Part model, mm, in its own coordinate system. Face numbers are marked on the shaded views. A direction names the side the tool comes from. Round coordinates to 2 decimals unless told otherwise and drop trailing zeros. Write each loop counter-clockwise with the first axis right and the second up, starting at its lowest first coordinate (ties: lowest second). Pieces come first, ordered by that corner, then holes.
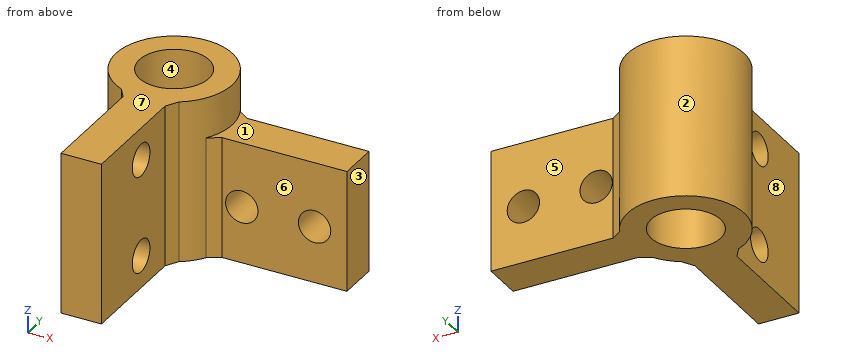
```python
from build123d import *

# Parameters (mm, degrees)
CYLINDER036_R          = 4.3
CYLINDER036_DEPTH      = 200
CYLINDER043_R          = 2
CYLINDER043_DEPTH      = 10
CYLINDER043_ROLL_ANGLE = 90
CYLINDER042_R          = 2
CYLINDER042_DEPTH      = 10
CYLINDER042_ROLL_ANGLE = 90
BOX010_W               = 24
BOX010_H               = 5
BOX010_DEPTH           = 15
CYLINDER044_R          = 2
CYLINDER044_DEPTH      = 10
CYLINDER045_R          = 2
CYLINDER045_DEPTH      = 10
BOX011_W               = 19
BOX011_H               = 5
BOX011_DEPTH           = 20
BOX011_PLACEMENT_ANGLE = -90
CYLINDER041_R          = 7.2
CYLINDER041_DEPTH      = 20
CHAMFER006_SIZE        = 1


with BuildPart() as cilindro033:
    # Cylinder036 → Cylinder036 (new body)
    with BuildSketch(Plane(origin=(57, -40, -29), x_dir=(1, 0, 0), z_dir=(0, 0, 1))):
        Circle(CYLINDER036_R)
    extrude(amount=CYLINDER036_DEPTH)


with BuildPart() as cilindro040:
    # Cylinder043 → Cylinder043 (new body)
    with BuildSketch(Plane.XY):
        Circle(CYLINDER043_R)
    extrude(amount=CYLINDER043_DEPTH)


with BuildPart() as cilindro040_1:
    # Cylinder043 roll: moved
    add(cilindro040.part.rotate(Axis((0, 0, 0), (1, 0, 0)), CYLINDER043_ROLL_ANGLE))


with BuildPart() as cilindro040_2:
    # Cylinder043 placement: moved
    add(cilindro040_1.part.moved(Location((76, -37, 30))))


with BuildPart() as fusion007:
    # Cylinder042 → Cylinder042 (new body)
    with BuildSketch(Plane.XY):
        Circle(CYLINDER042_R)
    extrude(amount=CYLINDER042_DEPTH)


with BuildPart() as fusion007_1:
    # Cylinder042 roll: moved
    add(fusion007.part.rotate(Axis((0, 0, 0), (1, 0, 0)), CYLINDER042_ROLL_ANGLE))


with BuildPart() as fusion007_2:
    # Cylinder042 placement: moved
    add(fusion007_1.part.moved(Location((67, -37, 30))))

    # Fusion007: union Cilindro040
    add(cilindro040_2.part)


with BuildPart() as cut032:
    # Box010 → Box010 (new body)
    with BuildSketch(Plane(origin=(56, -43, 23), x_dir=(1, 0, 0), z_dir=(0, 0, 1))):
        with Locations((12, 2.5)):
            Rectangle(BOX010_W, BOX010_H)
    extrude(amount=BOX010_DEPTH)

    # Cut032: cut Fusion007
    add(fusion007_2.part, mode=Mode.SUBTRACT)


with BuildPart() as cut032_1:
    # Cut032 placement: moved
    add(cut032.part.moved(Location((0, 0, -2))))


with BuildPart() as cilindro041:
    # Cylinder044 → Cylinder044 (new body)
    with BuildSketch(Plane(origin=(63, -53, 25), x_dir=(0, -1, 0), z_dir=(-1, 0, 0))):
        Circle(CYLINDER044_R)
    extrude(amount=CYLINDER044_DEPTH)


with BuildPart() as fusion008:
    # Cylinder045 → Cylinder045 (new body)
    with BuildSketch(Plane(origin=(63, -53, 37), x_dir=(0, -1, 0), z_dir=(-1, 0, 0))):
        Circle(CYLINDER045_R)
    extrude(amount=CYLINDER045_DEPTH)

    # Fusion008: union Cilindro041
    add(cilindro041.part)


with BuildPart() as cut033:
    # Box011 → Box011 (new body)
    with BuildSketch(Plane.XY):
        with Locations((9.5, 2.5)):
            Rectangle(BOX011_W, BOX011_H)
    extrude(amount=BOX011_DEPTH)


with BuildPart() as cut033_1:
    # Box011 placement: moved
    add(cut033.part.moved(Location((55, -43, 21))).rotate(Axis((55, -43, 21), (0, 0, 1)), BOX011_PLACEMENT_ANGLE))

    # Cut033: cut Fusion008
    add(fusion008.part, mode=Mode.SUBTRACT)


with BuildPart() as rodamiento_lineal:
    # Cylinder041 → Cylinder041 (new body)
    with BuildSketch(Plane(origin=(57, -40, 21), x_dir=(1, 0, 0), z_dir=(0, 0, 1))):
        Circle(CYLINDER041_R)
    extrude(amount=CYLINDER041_DEPTH)

    # Fusion009: union Cut032, Cut033
    add(cut032_1.part)
    add(cut033_1.part)

    # Chamfer006
    chamfer006_edges = [rodamiento_lineal.edges().sort_by_distance(p)[0] for p in [
        (63.916647, -38, 28.5),
        (63.545227, -43, 28.5),
        (55, -46.916647, 31),
        (60, -46.545227, 31),
    ]]
    chamfer(chamfer006_edges, length=CHAMFER006_SIZE)

    # Cut034: cut Cilindro033
    add(cilindro033.part, mode=Mode.SUBTRACT)


solid = rodamiento_lineal.part
```
Q1. Drop flat-ended pins along their axis: pin 1 (6 mm diameter, centred on x = 65, y = -53.5, fed in from -Z); pin 2 (7.5 mm diameter, centred on x = 71.5, z = 26.5, fed in from -Y); pin 3 (7.5 mm diameter, centred on x = 69.5, y = -41.5, fed in from +Z); pin 4 (5 mm diameter, centred on y = -53, z = 25, fed in from -X). Give the stop position or say it passes through.
Values follow:
pin 1: passes through
pin 2: stops at y = -43
pin 3: stops at z = 36
pin 4: stops at x = 55
Q2. Cut at A-A on y = -53. Write the cut outline in (x, z), plus the area to 3 significant figures.
Values follow:
outline: (55, 21) - (60, 21) - (60, 23) - (55, 23) - close; (55, 27) - (60, 27) - (60, 35) - (55, 35) - close; (55, 39) - (60, 39) - (60, 41) - (55, 41) - close
area: 60.0 mm2
Q3. Cut at B-B on x = 57. Write the cut outline in (y, z).
Values follow:
outline: (-62, 21) - (-44.3, 21) - (-44.3, 41) - (-62, 41) - close; (-35.7, 21) - (-32.8, 21) - (-32.8, 41) - (-35.7, 41) - close; hole circle Ø4 at (-53, 25); hole circle Ø4 at (-53, 37)
Q4. Cut at D-D on x = 76. Write the cut outline in (y, z), plus the area to 3 significant figures.
Values follow:
outline: (-43, 21) - (-38, 21) - (-38, 26) - (-43, 26) - close; (-43, 30) - (-38, 30) - (-38, 36) - (-43, 36) - close
area: 55.0 mm2
Q5. Which spindle directions (+Z, -Z, +X, -X, +Y, -Y) get a long thin tool onto all of the face, cutting with end or side? Do the marked faces 5, 6, 7 and 8. Say none if no direction does.
Values follow:
face 5: +Z, -Z, +X, +Y
face 6: +Z, -Z, +X, -Y
face 7: +Z, +X, -X, +Y, -Y
face 8: +Z, -Z, -X, -Y
Q6. Mould opens along X. For the marked faces 1, 2, 3 and 4 say: +X half, -X half, draft (parallel to the pull), parting line (faces both ways), or undercut.
Values follow:
face 1: draft
face 2: parting line
face 3: +X half
face 4: undercut
Q7. Cut at C-C on y = -41.75. Write the cut outline in (x, z).
Values follow:
outline: (50.02, 21) - (53.07, 21) - (53.07, 41) - (50.02, 41) - close; (60.93, 21) - (80, 21) - (80, 36) - (63.98, 36) - (63.98, 41) - (60.93, 41) - close; hole circle Ø4 at (67, 28); hole circle Ø4 at (76, 28)
Q8. Wall check: L1, parallel to Z at x = 58.95, y = -53; L2, parallel to X at y = -39.8, z = 28; L3, parallel to X at y = -41.8, z = 28. Give the ranges that are in metal, low to high.
Values follow:
L1: z = 21 to 23, 27 to 35, 39 to 41
L2: x = 49.8 to 52.7, 61.3 to 65, 69 to 74, 78 to 80
L3: x = 50.03 to 53.09, 60.91 to 65, 69 to 74, 78 to 80
